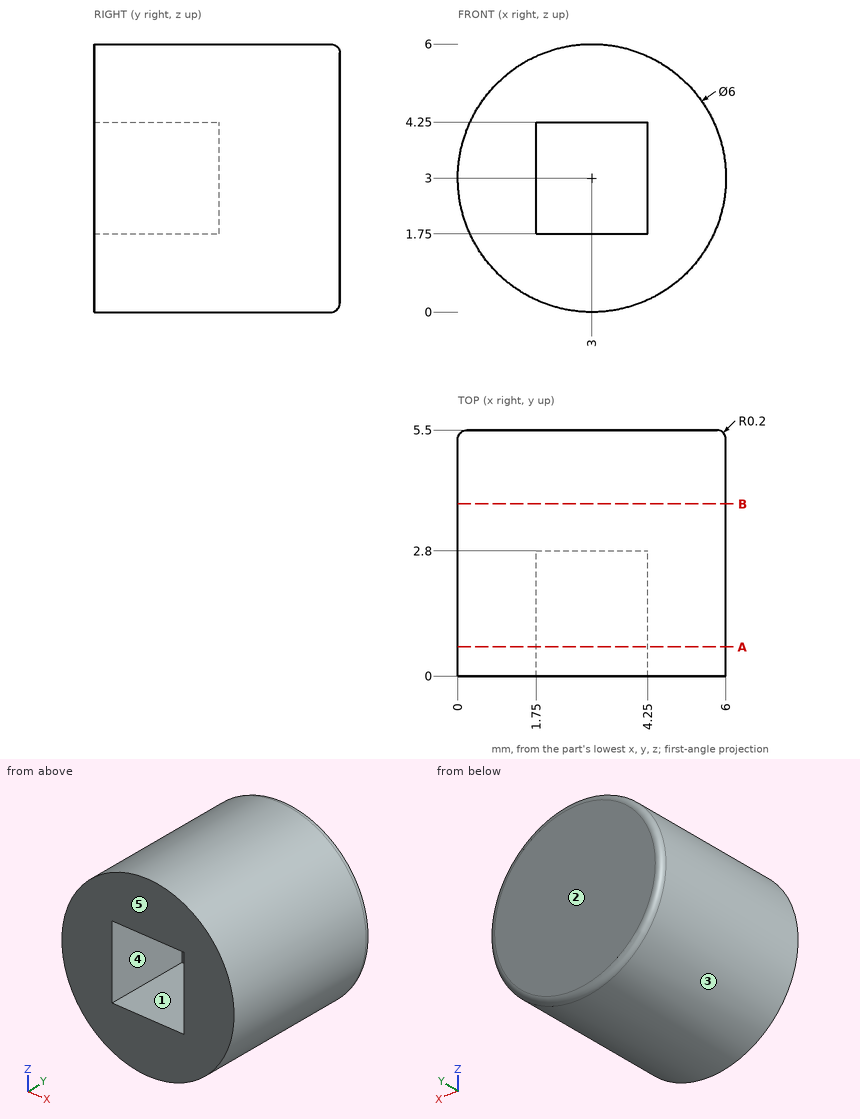
Here's the drawing with two shaded views (mm, measured from the low corner). I have some questions. A direction names the side the tool comes from. Coordinates: 2 decimals unless noted, no trailing zeros. Loops run counter-clockwise (first coordinate to the right, second up) from the corner with the lowest first, then second, coordinate; pieces in that order, holes last. Notation, with made-up numbers: M 76.25,79 L 128.25,79 A16 ccw 128.25,102 Z; hole C 85.5,84.5 d3. An arc over 180 degrees is marked long. Answer as CSV lines item,"result". Start each with the question number.
1. If I drill on probe 1 along Y at (x, z) = (2, 2.25); probe 2 along X at (y, z) = (0.8, 3.25); probe 3 along Z at (x, y) = (1.25, 4.1), over which ranges is the centre line in solid material (lowest first)? Write a range as [from, to].
2. Thinking about a two-plate mould opening in Z: for the marked faces 3, 4 and 5, which applies, +Z half, -Z half, draft (parallel to the pull), parting line (faces both ways), or undercut?
3. For pin 1 Ø1.5 at (y, z) = (2, 1.5) entering from -X; pin 2 Ø0.7 at (x, z) = (3, 2.5) entering from -Y, each with a flat end and sliding along its axis, tell me the tip position at first contact or that it passes through.
4. Suppose I cut it at A-A, the plane y = 0.65. List the corners of the cut face in (x, z) for me.
5. For the marked faces 1 and 2, which set-ups out of +Z, -Z, +X, -X, +Y, -Y let a thin tool reach every point of the face, with its end or its side?
6. Suppose I cut it at B-B, the plane y = 3.85. List the corners of the cut face in (x, z) for me, plus the area to 3 significant figures.
Output:
1,probe 1,"y = [2.8, 5.5]"
1,probe 2,"x = [0.01, 1.75], [4.25, 5.99]"
1,probe 3,"z = [0.56, 5.44]"
2,face 3,"parting line"
2,face 4,"undercut"
2,face 5,"draft"
3,pin 1,"stops at x = 0.1"
3,pin 2,"stops at y = 2.8"
4,outline,"C 3,3 d6; hole M 1.75,1.75 L 4.25,1.75 L 4.25,4.25 L 1.75,4.25 Z"
5,face 1,"-Y"
5,face 2,"+Z, -Z, +X, -X, +Y"
6,outline,"C 3,3 d6"
6,area,"28.3 mm^2"
